Input: dimensioned drawing with shaded views. Units: mm. Origin: part minimum x, y, z. Round coordinates to 2 decimals unless told otherwise and drop trailing zeros. Order: outer loops, then holes, each group sorted by start corner. A loop starts at its lowest first (then second) coordinate and runs counter-clockwise, first axis right, second up. Notation, with made-up numbers: M 56,22.25 L 62,22.25 A27 cw 62,45.25 Z; hole C -33,83.25 d6. An arc over 180 degrees is marked long. Answer as CSV lines item,"result". Start each with the question number.
Item 1: Section query C-C on y = 23. Return the cut outline in (x, z).
Item 2: Section query A-A on z = 17.5. Return the cut outline in (x, y).
Item 3: Pull-direction query (Y, two-part tool) for the marked faces 1, 2, 3 and 4; classes: +Y half, -Y half, draft (parallel to the pull), parting line (faces both ways), or undercut.
Item 4: Section query B-B on x = 17.5. Return the cut outline in (y, z).
Item 5: Line query: line 1 (Y direction, x = 6.5, z = 5.5); line 2 (X direction, y = 14.5, z = 17.5); line 3 (Z direction, x = 18.5, y = 5). Output: solid intervals per line, ascending. Write a range as [from, to].
Item 6: Section query D-D on z = 9.5. Return the cut outline in (x, y).
Item 7: First-contact query: P1, Ø6, axis at x = 29, y = 27, coming from the -Z side; P2, Ø3, axis at y = 18.5, z = 19, coming from the +X side; P3, Ø12, axis at x = 31, y = 18.5, coming from the +Z side; P4, Ø5, axis at x = 17.5, z = 17.5, coming from the -Y side. Flat tips, straight axial feed; report the tip coordinate or a pass-through.
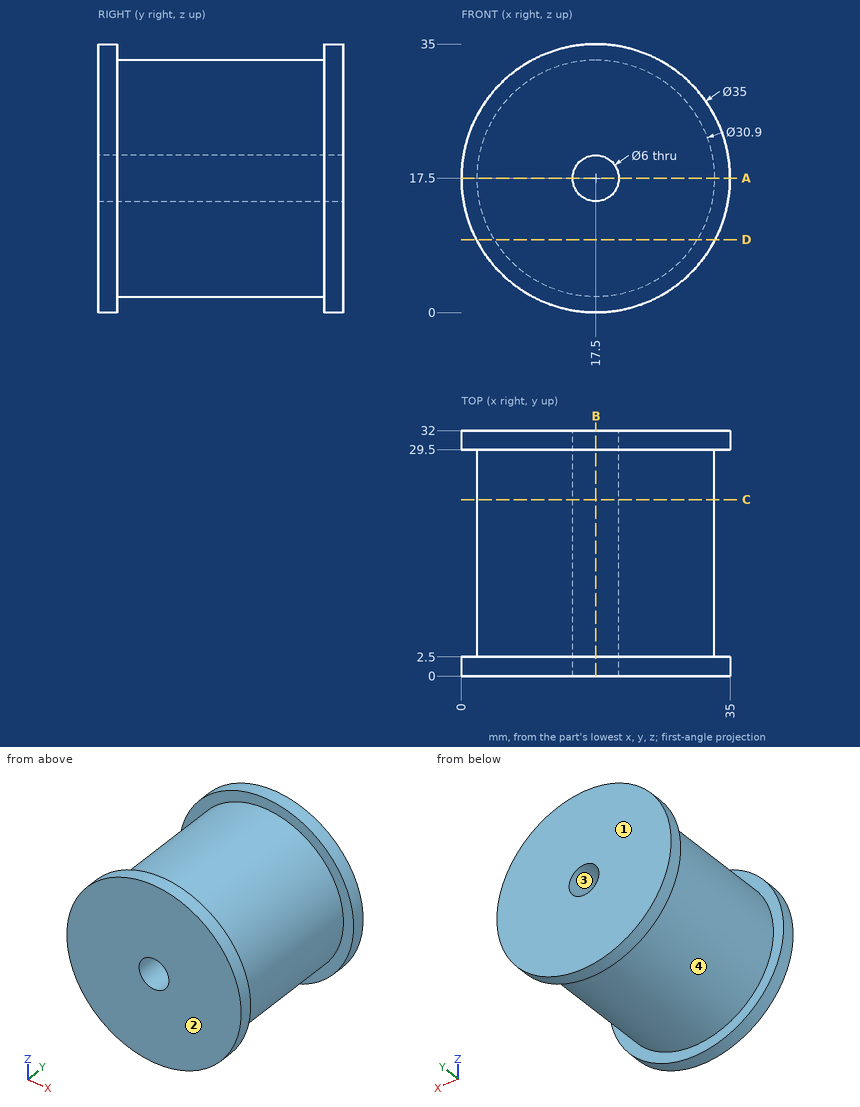
Results:
1,outline,"C 17.5,17.5 d30.9; hole C 17.5,17.5 d6"
2,outline,"M 0,0 L 14.5,0 L 14.5,32 L 0,32 L 0,29.5 L 2.05,29.5 L 2.05,2.5 L 0,2.5 Z; M 20.5,0 L 35,0 L 35,2.5 L 32.95,2.5 L 32.95,29.5 L 35,29.5 L 35,32 L 20.5,32 Z"
3,face 1,"+Y half"
3,face 2,"-Y half"
3,face 3,"draft"
3,face 4,"undercut"
4,outline,"M 0,0 L 2.5,0 L 2.5,2.05 L 29.5,2.05 L 29.5,0 L 32,0 L 32,14.5 L 0,14.5 Z; M 0,20.5 L 32,20.5 L 32,35 L 29.5,35 L 29.5,32.95 L 2.5,32.95 L 2.5,35 L 0,35 Z"
5,line 1,"[0, 2.5], [29.5, 32]"
5,line 2,"[2.05, 14.5], [20.5, 32.95]"
5,line 3,"[2.08, 14.67], [20.33, 32.92]"
6,outline,"M 1.94,0 L 33.06,0 L 33.06,2.5 L 30.72,2.5 L 30.72,29.5 L 33.06,29.5 L 33.06,32 L 1.94,32 L 1.94,29.5 L 4.28,29.5 L 4.28,2.5 L 1.94,2.5 Z"
7,P1,"z = 3.03"
7,P2,"x = 32.95"
7,P3,"z = 31.01"
7,P4,"through"
